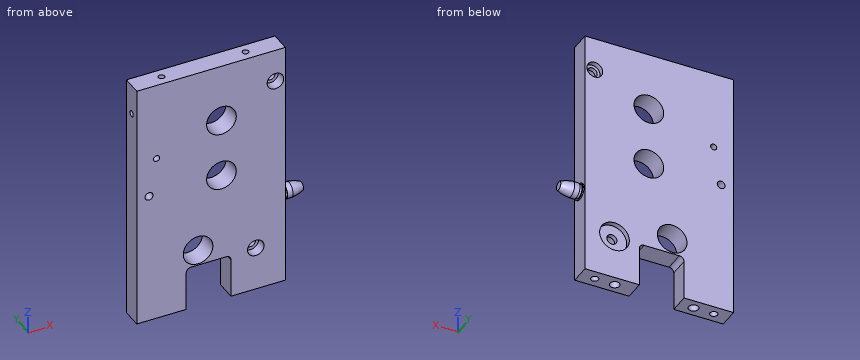
from build123d import *

# Parameters (mm, degrees)
SKETCH1_W           = 95.25
SKETCH1_H           = 12.8
BOSS_EXTRUDE1_DEPTH = 161.88
SKETCH1_3_R         = 3.1
CUT_EXTRUDE1_DEPTH  = 20.2
SKETCH1_4_R         = 2.395
CUT_EXTRUDE2_DEPTH  = 21.5
CUT_EXTRUDE3_REACH  = 14.8
SKETCH2_R           = 9.525
CUT_EXTRUDE4_REACH  = 14.8
SKETCH3_R           = 3.265
SKETCH3_R_2         = 1.96
SKETCH3_R_3         = 2.56
SKETCH4_R           = 9.525
SKETCH4_R_2         = 5.09
CUT_EXTRUDE5_DEPTH  = 3.32
SKETCH5_R           = 5.31
CUT_EXTRUDE6_DEPTH  = 6.65
SKETCH6_R           = 1.965
CUT_EXTRUDE7_DEPTH  = 17.25
SKETCH7_R           = 1.97
CUT_EXTRUDE8_DEPTH  = 15.87
SKETCH9_R           = 9.5
CUT_EXTRUDE9_DEPTH  = 13.8000001


with BuildPart() as part:
    # Sketch1 → Boss-Extrude1 (new body)
    with BuildSketch(Plane.XY):
        with Locations((-282.25, -616.5)):
            Rectangle(SKETCH1_W, SKETCH1_H)
    extrude(amount=BOSS_EXTRUDE1_DEPTH)

    # Sketch1_3 → Cut-Extrude1 (cut)
    with BuildSketch(Plane.XY):
        with Locations((-307.5, -616.5)):
            Circle(SKETCH1_3_R)
        with Locations((-257, -616.5)):
            Circle(SKETCH1_3_R)
    extrude(amount=CUT_EXTRUDE1_DEPTH, mode=Mode.SUBTRACT)

    # Sketch1_4 → Cut-Extrude2 (cut)
    with BuildSketch(Plane.XY):
        with Locations((-244.2, -616.5)):
            Circle(SKETCH1_4_R)
        with Locations((-320.5, -616.5)):
            Circle(SKETCH1_4_R)
    extrude(amount=CUT_EXTRUDE2_DEPTH, mode=Mode.SUBTRACT)

    # Sketch2 → Cut-Extrude3 (cut, up to next)
    with BuildSketch(Plane(origin=(0, -610.1, 0), x_dir=(1, 0, 0), z_dir=(0, 1, 0)), mode=Mode.PRIVATE) as cut_extrude3_sk1:
        with Locations((-275.57, -124.135)):
            Circle(SKETCH2_R)
    cut_extrude3_tool1 = extrude(cut_extrude3_sk1.sketch, amount=-CUT_EXTRUDE3_REACH, mode=Mode.PRIVATE) & part.part
    add(cut_extrude3_tool1.solids().sort_by_distance((-275.57, -610.1, 124.135))[0], mode=Mode.SUBTRACT)
    # Sketch2 → Cut-Extrude3 (cut, up to next)
    with BuildSketch(Plane(origin=(0, -610.1, 0), x_dir=(1, 0, 0), z_dir=(0, 1, 0)), mode=Mode.PRIVATE) as cut_extrude3_sk2:
        with Locations((-275.57, -86.105)):
            Circle(SKETCH2_R)
    cut_extrude3_tool2 = extrude(cut_extrude3_sk2.sketch, amount=-CUT_EXTRUDE3_REACH, mode=Mode.PRIVATE) & part.part
    add(cut_extrude3_tool2.solids().sort_by_distance((-275.57, -610.1, 86.105))[0], mode=Mode.SUBTRACT)
    # Sketch2 → Cut-Extrude3 (cut, up to next)
    with BuildSketch(Plane(origin=(0, -610.1, 0), x_dir=(1, 0, 0), z_dir=(0, 1, 0)), mode=Mode.PRIVATE) as cut_extrude3_sk3:
        with BuildLine():
            Line((-269.505, 0), (-298.155, 0))
            Line((-298.155, 0), (-298.155, -25.4))
            ThreePointArc((-298.155, -25.4), (-297.276320344, -27.521320344), (-295.155, -28.4))
            Line((-295.155, -28.4), (-272.505, -28.4))
            ThreePointArc((-272.505, -28.4), (-270.383679656, -27.521320344), (-269.505, -25.4))
            Line((-269.505, -25.4), (-269.505, 0))
        make_face()
    cut_extrude3_tool3 = extrude(cut_extrude3_sk3.sketch, amount=-CUT_EXTRUDE3_REACH, mode=Mode.PRIVATE) & part.part
    add(cut_extrude3_tool3.solids().sort_by_distance((-283.83, -610.1, 14.135461))[0], mode=Mode.SUBTRACT)

    # Sketch3 → Cut-Extrude4 (cut, up to next)
    with BuildSketch(Plane(origin=(0, -610.1, 0), x_dir=(-1, 0, 0), z_dir=(0, 1, 0)), mode=Mode.PRIVATE) as cut_extrude4_sk1:
        with Locations((240.925, 140.49)):
            Circle(SKETCH3_R)
    cut_extrude4_tool1 = extrude(cut_extrude4_sk1.sketch, amount=-CUT_EXTRUDE4_REACH, mode=Mode.PRIVATE) & part.part
    add(cut_extrude4_tool1.solids().sort_by_distance((-240.925, -610.1, 140.49))[0], mode=Mode.SUBTRACT)
    # Sketch3 → Cut-Extrude4 (cut, up to next)
    with BuildSketch(Plane(origin=(0, -610.1, 0), x_dir=(-1, 0, 0), z_dir=(0, 1, 0)), mode=Mode.PRIVATE) as cut_extrude4_sk2:
        with Locations((253.55, 28.505)):
            Circle(SKETCH3_R)
    cut_extrude4_tool2 = extrude(cut_extrude4_sk2.sketch, amount=-CUT_EXTRUDE4_REACH, mode=Mode.PRIVATE) & part.part
    add(cut_extrude4_tool2.solids().sort_by_distance((-253.55, -610.1, 28.505))[0], mode=Mode.SUBTRACT)
    # Sketch3 → Cut-Extrude4 (cut, up to next)
    with BuildSketch(Plane(origin=(0, -610.1, 0), x_dir=(-1, 0, 0), z_dir=(0, 1, 0)), mode=Mode.PRIVATE) as cut_extrude4_sk3:
        with Locations((317.175, 111.08)):
            Circle(SKETCH3_R_2)
    cut_extrude4_tool3 = extrude(cut_extrude4_sk3.sketch, amount=-CUT_EXTRUDE4_REACH, mode=Mode.PRIVATE) & part.part
    add(cut_extrude4_tool3.solids().sort_by_distance((-317.175, -610.1, 111.08))[0], mode=Mode.SUBTRACT)
    # Sketch3 → Cut-Extrude4 (cut, up to next)
    with BuildSketch(Plane(origin=(0, -610.1, 0), x_dir=(-1, 0, 0), z_dir=(0, 1, 0)), mode=Mode.PRIVATE) as cut_extrude4_sk4:
        with Locations((321.975, 86.28)):
            Circle(SKETCH3_R_3)
    cut_extrude4_tool4 = extrude(cut_extrude4_sk4.sketch, amount=-CUT_EXTRUDE4_REACH, mode=Mode.PRIVATE) & part.part
    add(cut_extrude4_tool4.solids().sort_by_distance((-321.975, -610.1, 86.28))[0], mode=Mode.SUBTRACT)

    # Sketch4 → Cut-Extrude5 (cut)
    with BuildSketch(Plane(origin=(0, -610.1, 0), x_dir=(-1, 0, 0), z_dir=(0, 1, 0))):
        with Locations((253.55, 28.505)):
            Circle(SKETCH4_R)
        with Locations((240.925, 140.49)):
            Circle(SKETCH4_R_2)
    extrude(amount=-CUT_EXTRUDE5_DEPTH, mode=Mode.SUBTRACT)

    # Sketch5 → Cut-Extrude6 (cut)
    with BuildSketch(Plane.XZ.offset(622.9)):
        with Locations((-240.925, 140.49)):
            Circle(SKETCH5_R)
        with Locations((-253.55, 28.505)):
            Circle(SKETCH5_R)
    extrude(amount=-CUT_EXTRUDE6_DEPTH, mode=Mode.SUBTRACT)

    # Sketch6 → Cut-Extrude7 (cut)
    with BuildSketch(Plane.XY.offset(161.88)):
        with Locations((-310.715, -616.48)):
            Circle(SKETCH6_R)
        with Locations((-256.825, -616.48)):
            Circle(SKETCH6_R)
    extrude(amount=-CUT_EXTRUDE7_DEPTH, mode=Mode.SUBTRACT)

    # Sketch7 → Cut-Extrude8 (cut)
    with BuildSketch(Plane.ZY.offset(329.875)):
        with Locations((142.28, -616.5)):
            Circle(SKETCH7_R)
    extrude(amount=-CUT_EXTRUDE8_DEPTH, mode=Mode.SUBTRACT)

    # Sketch8 → Revolve1 (revolve)
    with BuildSketch(Plane(origin=(0, -616.5, 0), x_dir=(-1, 0, 0), z_dir=(0, 1, 0))):
        with BuildLine():
            Line((234.625, 57.29), (221.025, 57.29))
            Line((221.025, 57.29), (221.025, 54.59))
            ThreePointArc((221.025, 54.59), (224.841543887, 53.18542762), (228.845807042, 52.475))
            Line((228.845807042, 52.475), (232.275807042, 52.475))
            Line((232.275807042, 52.475), (232.295, 52.925))
            Line((232.295, 52.925), (233.835, 52.925))
            Line((233.835, 52.925), (233.835, 52.09))
            Line((233.835, 52.09), (234.625, 52.09))
            Line((234.625, 52.09), (234.625, 57.29))
        make_face()
    revolve(axis=Axis((-234.625, -616.5, 57.29), (-1, 0, 0)))

    # Sketch9 → Cut-Extrude9 (cut, through all)
    with BuildSketch(Plane.XZ.offset(622.9)):
        with Locations((-290.57, 38.77)):
            Circle(SKETCH9_R)
    extrude(amount=-CUT_EXTRUDE9_DEPTH, mode=Mode.SUBTRACT)


solid = part.part
Design review of the part built by this model. Coordinates are the model's own, in mm. Give positions to 0.01 mm unless a question says otherwise; leave off trailing zeros. Loops run counter-clockwise (first coordinate to the right, second up) from the corner with the lowest first, then second, coordinate; pieces in that order, holes last. Notation, with made-up numbers: (70.5, 81) -> (118.5, 81) arc R27 ccw to (118.5, 109) -> close; hole circle Ø8 at (-6, -7.75). An arc over 180 degrees is marked (long way). One line per question, with ' | ' between items. Start each with the question number.
(1) We need section C-C (x = -275.57). State the section outline as (y, z) points.
(2) We need section D-D (z = 66). State the section outline as (x, y) points (3 decimals).
(3) We need section B-B (x = -290.57). State the section outline as (y, z) points.
(4) Insertion check: P1, Ø2.5, axis at x = -310.715, y = -616.48, coming from the +Z side; P2, Ø1.4, axis at x = -320.5, y = -616.5, coming from the -Z side; P3, Ø12, axis at x = -253.55, z = 28.505, coming from the +Y side; P4, Ø17, axis at x = -275.57, z = 86.105, coming from the +Y side. Each pin has a flat end and moves straight along its axis. Give the tip position at first contact, or say it passes through.
(5) For line 1 (X direction, y = -616.5, z = 13.75) (3 decimals); line 2 (X direction, y = -611.25, z = 26) (3 decimals); line 3 (Z direction, x = -273, y = -614.5), list the stretches that pass through material, from the lowest coordinate up.
(6) We need section A-A (z = 111.08). State the section outline as (x, y) points (3 decimals).
The answers:
1) outline: (-622.9, 28.4) -> (-610.1, 28.4) -> (-610.1, 76.58) -> (-622.9, 76.58) -> close; (-622.9, 95.63) -> (-610.1, 95.63) -> (-610.1, 114.61) -> (-622.9, 114.61) -> close; (-622.9, 133.66) -> (-610.1, 133.66) -> (-610.1, 161.88) -> (-622.9, 161.88) -> close
2) outline: (-329.875, -622.9) -> (-234.625, -622.9) -> (-234.625, -610.1) -> (-329.875, -610.1) -> close
3) outline: (-622.9, 28.4) -> (-610.1, 28.4) -> (-610.1, 29.27) -> (-622.9, 29.27) -> close; (-622.9, 48.27) -> (-610.1, 48.27) -> (-610.1, 161.88) -> (-622.9, 161.88) -> close
4) P1: stops at z = 144.63 | P2: stops at z = 21.5 | P3: stops at y = -613.42 | P4: passes through
5) line 1: x = -329.875 to -322.895, -318.105 to -310.6, -304.4 to -298.155, -269.505 to -260.1, -253.9 to -246.595, -241.805 to -234.625 | line 2: x = -329.875 to -298.094, -269.566 to -262.74, -244.36 to -234.625 | line 3: z = 28.4 to 76.93, 95.28 to 114.96, 133.31 to 161.88
6) outline: (-329.875, -622.9) -> (-319.135, -622.9) -> (-319.135, -610.1) -> (-329.875, -610.1) -> close; (-315.215, -622.9) -> (-234.625, -622.9) -> (-234.625, -610.1) -> (-315.215, -610.1) -> close
